Design review of the part shown in the three views and the two pictorial views. Dimensions are in mm from the part's minimum x, y and z. Coordinates: 2 decimals unless noted, no trailing zeros. Write each loop counter-clockwise with the first axis right and the second up, starting at its lowest first coordinate (ties: lowest second). Pieces come first, ordered by that corner, then holes. Notation, with made-up numbers: M 51,-35.75 L 84,-35.75 A29 ccw 84,-11.75 Z; hole C -32,-17 d2. An arc over 180 degrees is marked long. Answer as a JSON object with one key per item and string values.
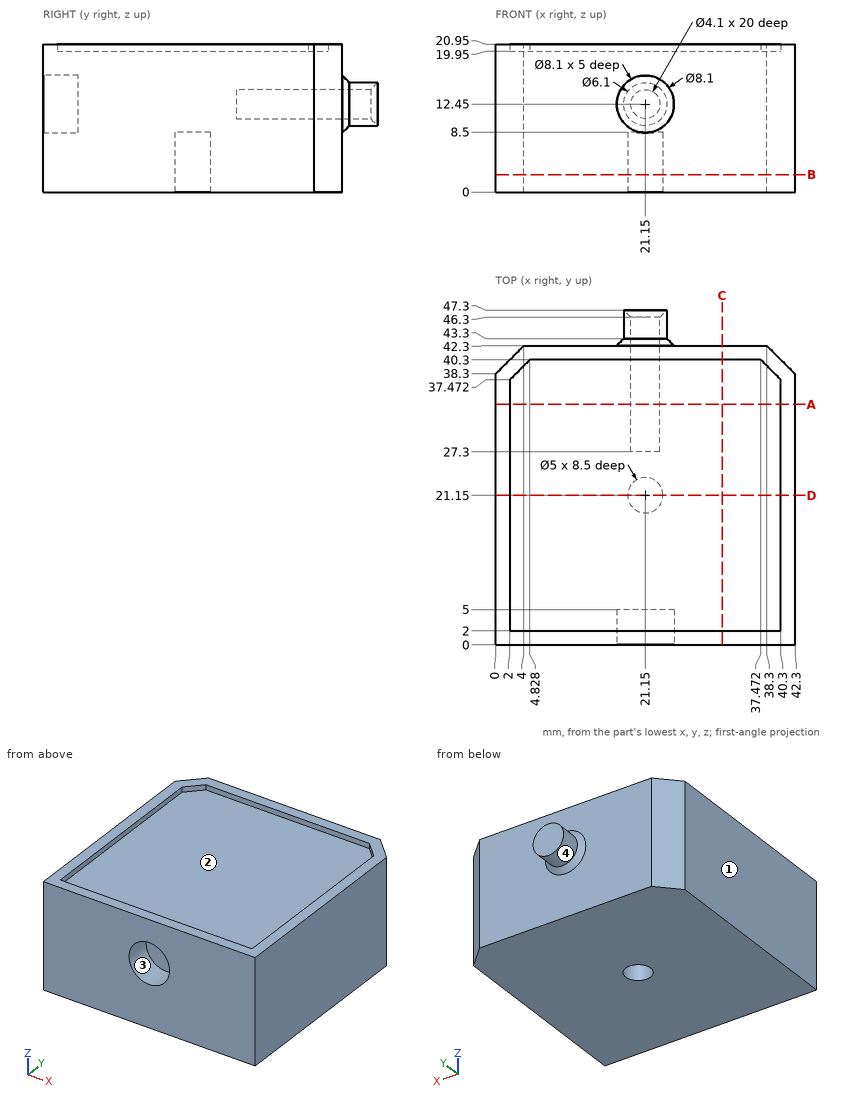
(1) Draft analysis for pull direction Z (two halves, no side actions). For the marked faces 1, 2, 3 and 4, state which applies: released by +Z, released by -Z, zero draft, split by the parting line, or undercut.
Results list:
{"face 1": "zero draft", "face 2": "released by +Z", "face 3": "undercut", "face 4": "split by the parting line"}
(2) Wall thickness on line 1 along Z through (x, y) = (21, 3); line 2 along X through (y, z) = (32, 12.45); line 3 along Z through (x, y) = (39.5, 24): over which ranges is each line inside the solid? List them lowest first. Write a range as from..to.
Results list:
{"line 1": "0..8.4, 16.5..19.95", "line 2": "0..19.1, 23.2..42.3", "line 3": "0..19.95"}
(3) Add section D-D on y = 21.15. Give the boundary of the cut face in (x, z).
Results list:
{"outline": "M 0,0 L 18.65,0 L 18.65,8.5 L 23.65,8.5 L 23.65,0 L 42.3,0 L 42.3,20.95 L 40.3,20.95 L 40.3,19.95 L 2,19.95 L 2,20.95 L 0,20.95 Z"}
(4) Add section C-C on x = 32. Give the boundary of the cut face in (y, z), and give its area (3 significant figures).
Results list:
{"outline": "M 0,0 L 42.3,0 L 42.3,20.95 L 40.3,20.95 L 40.3,19.95 L 2,19.95 L 2,20.95 L 0,20.95 Z", "area": "848 mm²"}
(5) For pin 1 Ø1.2 at (x, z) = (20.5, 11.5) entering from +Y; pin 2 Ø5 at (x, z) = (21.15, 12.45) entering from -Y; pin 3 Ø1.5 at (x, z) = (18.5, 6.5) entering from +Y, all flat-tipped, find the tip position at first contact; note any pin that passes through.
Results list:
{"pin 1": "y = 27.3", "pin 2": "y = 5", "pin 3": "y = 42.3"}
(6) Add section A-A on y = 34. Give the boundary of the cut face in (x, z), and give its area (3 significant figures).
Results list:
{"outline": "M 0,0 L 42.3,0 L 42.3,20.95 L 40.3,20.95 L 40.3,19.95 L 2,19.95 L 2,20.95 L 0,20.95 Z; hole C 21.15,12.45 d4.1", "area": "835 mm²"}
(7) Add section B-B on z = 2.5. Give the boundary of the cut face in (x, y), and give its area (3 significant figures).
Results list:
{"outline": "M 0,0 L 42.3,0 L 42.3,38.3 L 38.3,42.3 L 4,42.3 L 0,38.3 Z; hole C 21.15,21.15 d5", "area": "1,750 mm²"}
